Autodesk Inventor part; units mm, degrees
ref_plane "YZ Plane" through (0, 0, 0) normal (1, 0, 0) x (0, 1, 0)
ref_plane "XZ Plane" through (0, 0, 0) normal (0, 1, 0) x (-1, 0, 0)
ref_plane "XY Plane" through (0, 0, 0) normal (0, 0, 1) x (1, 0, 0)
sketch "Sketch6" plane through (0, 0, 0) normal (0, 0, 1) x (1, 0, 0)
  line L0 (0, 0) -> (130, 0)
  line L1 (130, 0) -> (130, 130)
  line L2 (130, 130) -> (0, 130)
  line L3 (0, 130) -> (0, 0)
  circle A0 centre (65, 65) radius 42.5
  dimension "d28" = 130
  dimension "d29" = 130
  dimension "d30" = 85
  dimension "d31" = 65
  dimension "d32" = 65
extrude "Extrusion6" add sketch "Sketch6" along normal blind 37
sketch "Sketch7" plane through (0, 0, 37) normal (0, 0, 1) x (1, 0, 0)
  circle A0 centre (116.265, 116.265) radius 4.5
  line L0 (130, 0) -> (130, 130)
  circle A1 centre (65, 65) radius 42.5
  circle A2 centre (13.735, 116.265) radius 4.5
  circle A3 centre (13.735, 13.735) radius 4.5
  circle A4 centre (116.265, 13.735) radius 4.5
  point P0 (0, 0)
  dimension "d36" = 51.265
  dimension "d37" = 51.265
  dimension "d38" = 9
  dimension "d39" = 9
  dimension "d40" = 9
  dimension "d41" = 9
  dimension "d42" = 51.265
  dimension "d43" = 51.265
  dimension "d44" = 51.265
  dimension "d45" = 51.265
  dimension "d46" = 51.265
  dimension "d47" = 51.265
extrude "Extrusion7" cut sketch "Sketch7" against normal blind 37 contours A0 | A2 | A3 | A4
fillet "Fillet1" radius 15 4 edges at (0, 130, 18.5) (130, 130, 18.5) (130, 0, 18.5) (0, 0, 18.5)
sketch "Sketch9" plane through (0, 0, 0) normal (0, 0, -1) x (-1, 0, 0)
  circle A0 centre (-65, 65) radius 42.5
  circle A1 centre (-65, 65) radius 42.5
  circle A2 centre (-65, 65) radius 22.5
  point P0 (0, 0)
  dimension "d54" = 85
  dimension "d55" = 45
extrude "Extrusion9" add sketch "Sketch9" against normal blind 18
sketch "Sketch10" plane through (0, 0, 0) normal (0, 0, -1) x (-1, 0, 0)
  circle A0 centre (-65, 65) radius 22.5
  circle A1 centre (-65, 65) radius 55
  point P0 (0, 0)
  dimension "d58" = 110
extrude "Extrusion10" cut sketch "Sketch10" against normal blind 6
equation "\"d31\" = 0.5 * d28"
equation "\"d32\" = 0.5 * d29"
equation "\"d42\" = d36"
equation "\"d43\" = d36"
equation "\"d44\" = d36"
equation "\"d45\" = d36"
equation "\"d46\" = d36"
equation "\"d47\" = d36"
properties part number "EndEffectorMotorAdapter"
Design review of the part built by this model. Coordinates are the model's own, in mm. A direction names the side the tool comes from. Round coordinates to 2 decimals unless told otherwise and drop trailing zeros. Loops run counter-clockwise (first coordinate to the right, second up) from the corner with the lowest first, then second, coordinate; pieces in that order, holes last. Notation, with made-up numbers: (-34.5, 36) - (-20.5, 36) arc R10 cw to (-20.5, 48) - close; hole circle Ø1 at (12, 13.25). An arc over 180 degrees is marked (long way). One line per question, with ' | ' between items.
1. For L1, parallel to Y at x = 15, z = 3; L2, parallel to X at y = 26, z = 29.5; L3, parallel to X at y = 53, z = 7, list the stretches that pass through material, from the lowest coordinate up. Write a range as [from, to].
Results are:
L1: y = [0, 9.42], [18.05, 42.09], [87.91, 111.95], [120.58, 130] | L2: x = [0, 48.11], [81.89, 130] | L3: x = [0, 45.97], [84.03, 130]
2. We need section C-C, the plane z = 33.5. State the section outline as (x, y) points (3 decimals), and give its area (3 significant figures).
Results are:
outline: (0, 15) arc R15 ccw to (15, 0) - (115, 0) arc R15 ccw to (130, 15) - (130, 115) arc R15 ccw to (115, 130) - (15, 130) arc R15 ccw to (0, 115) - close; hole circle Ø9 at (13.735, 13.735); hole circle Ø9 at (13.735, 116.265); hole circle Ø85 at (65, 65); hole circle Ø9 at (116.265, 13.735); hole circle Ø9 at (116.265, 116.265) | area: 10,800 mm²
3. We need section A-A, the plane y = 65. State the section outline as (x, z) points, and give its area (4 significant figures).
Results are:
outline: (0, 0) - (10, 0) - (10, 6) - (42.5, 6) - (42.5, 18) - (22.5, 18) - (22.5, 37) - (0, 37) - close; (87.5, 6) - (120, 6) - (120, 0) - (130, 0) - (130, 37) - (107.5, 37) - (107.5, 18) - (87.5, 18) - close | area: 1,995 mm²
4. We need section B-B, the plane x = 83. State the section outline as (y, z) points.
Results are:
outline: (0, 0) - (13.03, 0) - (13.03, 6) - (51.5, 6) - (51.5, 18) - (26.5, 18) - (26.5, 37) - (0, 37) - close; (78.5, 6) - (116.97, 6) - (116.97, 0) - (130, 0) - (130, 37) - (103.5, 37) - (103.5, 18) - (78.5, 18) - close
5. Draft analysis for pull direction Y (two halves, no side actions). For faces 4 (the face through (64, 0, 18)), 5 (the face through (64, 109, 37)), 6 (the face through (81.58, 80.21, 11.92)), state which applies: released by +Y, released by -Y, zero draft, split by the parting line, or undercut.
Results are:
face 4: released by -Y | face 5: zero draft | face 6: undercut
6. We need section D-D, the plane x = 27.5. State the section outline as (y, z) points, and give its area (3 significant figures).
Results are:
outline: (0, 0) - (24.77, 0) - (24.77, 6) - (105.23, 6) - (105.23, 0) - (130, 0) - (130, 37) - (85, 37) - (85, 18) - (45, 18) - (45, 37) - (0, 37) - close | area: 3,570 mm²
7. For faces 1 (the face through (13.149, 120.727, 18.759)), 2 (the face through (47, 47, 18)), 3 (the face through (66, 41, 6)), list the 3-axis set-ups (+Z, -Z, +X, -X, +Y, -Y) from which the entire face can be reached by the end or side of a thin tool; tool diameter is ignored.
Results are:
face 1: +Z, -Z | face 2: +Z | face 3: -Z
